Source: CAD feature listing. Evaluate the final solid. Frame: model axes, mm. A direction names the side the tool comes from. Round coordinates to 2 decimals unless told otherwise and drop trailing zeros. Loops run counter-clockwise (first coordinate to the right, second up) from the corner with the lowest first, then second, coordinate; pieces in that order, holes last. Notation, with made-up numbers: M 60.5,4.25 L 81.5,4.25 A14 cw 81.5,27.25 Z; hole C 2,33.5 d3. An arc over 180 degrees is marked long. Answer as a JSON object with one key per item and string values.
from build123d import *

# Parameters (mm, degrees)
F1_DEPTH = 6.35
F2_R     = 2.9845
F3_DEPTH = 6.35
F4_R     = 5.08
F5_R     = 3.81


with BuildPart() as f1:
    # F0 (on Top) → F1 (new body)
    with BuildSketch(Plane.XY):
        with BuildLine():
            Line((-10.9985226281, 6.35), (10.9985226281, 6.35))
            ThreePointArc((10.9985226281, 6.35), (0, 12.7), (-10.9985226281, 6.35))
        make_face()
        with BuildLine():
            ThreePointArc((-10.9985226281, -6.35), (-12.7, 0), (-10.9985226281, 6.35))
            Line((-10.9985226281, 6.35), (-31.75, 6.35))
            Line((-31.75, 6.35), (-31.75, -6.35))
            Line((-31.75, -6.35), (-10.9985226281, -6.35))
        make_face()
        with BuildLine():
            ThreePointArc((10.9985226281, -6.35), (12.2672579939, -3.2870018728), (12.7, 0))
            ThreePointArc((12.7, 0), (12.2672579939, 3.2870018728), (10.9985226281, 6.35))
            Line((10.9985226281, 6.35), (-10.9985226281, 6.35))
            ThreePointArc((-10.9985226281, 6.35), (-12.7, 0), (-10.9985226281, -6.35))
            Line((-10.9985226281, -6.35), (10.9985226281, -6.35))
        make_face()
        with BuildLine():
            ThreePointArc((10.9985226281, 6.35), (12.2672579939, 3.2870018728), (12.7, 0))
            ThreePointArc((12.7, 0), (12.2672579939, -3.2870018728), (10.9985226281, -6.35))
            Line((10.9985226281, -6.35), (31.75, -6.35))
            Line((31.75, -6.35), (31.75, 6.35))
            Line((31.75, 6.35), (10.9985226281, 6.35))
        make_face()
        with BuildLine():
            ThreePointArc((-10.9985226281, -6.35), (0, -12.7), (10.9985226281, -6.35))
            Line((10.9985226281, -6.35), (-10.9985226281, -6.35))
        make_face()
    extrude(amount=F1_DEPTH)

    # F2 (on face) → F3 (cut)
    with BuildSketch(Plane.XY.offset(6.35)):
        Circle(F2_R)
    extrude(amount=-F3_DEPTH, mode=Mode.SUBTRACT)

    # F4
    f4_edges = [f1.edges().sort_by_distance(p)[0] for p in [
        (-10.998523, 6.35, 3.175),
        (10.998523, -6.35, 3.175),
        (-10.998523, -6.35, 3.175),
        (10.998523, 6.35, 3.175),
    ]]
    fillet(f4_edges, radius=F4_R)

    # F5
    f5_edges = [f1.edges().sort_by_distance(p)[0] for p in [
        (-31.75, 6.35, 3.175),
        (-31.75, -6.35, 3.175),
        (31.75, -6.35, 3.175),
        (31.75, 6.35, 3.175),
    ]]
    fillet(f5_edges, radius=F5_R)


solid = f1.part
Item 1: Contact query for flat-ended pins moving along their axis: pin 1 Ø1.5 at (y, z) = (5.5, 4.5) entering from -X; pin 2 Ø1 at (x, y) = (-8, -9.5) entering from -Z; pin 3 Ø1 at (y, z) = (6, 4.5) entering from -X; pin 4 Ø3 at (x, z) = (15, 4.5) entering from +Y. Output: stop coordinate, or through.
Answer sheet:
{"pin 1": "stops at x = -31.04", "pin 2": "stops at z = 0", "pin 3": "stops at x = -30.34", "pin 4": "stops at y = 6.35"}
Item 2: Section A-A on z = 4.5. Return the cut outline in (x, y).
Answer sheet:
{"outline": "M -31.75,-2.54 A3.81 ccw -27.94,-6.35 L -13.62,-6.35 A5.08 cw -9.73,-8.16 A12.7 ccw 9.73,-8.16 A5.08 cw 13.62,-6.35 L 27.94,-6.35 A3.81 ccw 31.75,-2.54 L 31.75,2.54 A3.81 ccw 27.94,6.35 L 13.62,6.35 A5.08 cw 9.73,8.16 A12.7 ccw -9.73,8.16 A5.08 cw -13.62,6.35 L -27.94,6.35 A3.81 ccw -31.75,2.54 Z; hole C 0,0 d5.97"}
Item 3: Section C-C on y = 1.75. Return the cut outline in (x, z).
Answer sheet:
{"outline": "M -31.75,0 L -2.42,0 L -2.42,6.35 L -31.75,6.35 Z; M 2.42,0 L 31.75,0 L 31.75,6.35 L 2.42,6.35 Z"}
Item 4: Section B-B on x = 0. Return the cut outline in (y, z), then the cut area to 3 significant figures.
Answer sheet:
{"outline": "M -12.7,0 L -2.98,0 L -2.98,6.35 L -12.7,6.35 Z; M 2.98,0 L 12.7,0 L 12.7,6.35 L 2.98,6.35 Z", "area": "123 mm²"}
Item 5: Section D-D on x = -22. Return the cut outline in (y, z).
Answer sheet:
{"outline": "M -6.35,0 L 6.35,0 L 6.35,6.35 L -6.35,6.35 Z"}
Item 6: Line query: probe 1 along Y at (x, z) = (0, 2); probe 2 along Y at (x, z) = (-18, 3.5); probe 3 along Y at (x, z) = (1, 1.5). Output: solid intervals per line, ascending. Write a range as from..to.
Answer sheet:
{"probe 1": "y = -12.7..-2.98, 2.98..12.7", "probe 2": "y = -6.35..6.35", "probe 3": "y = -12.66..-2.81, 2.81..12.66"}
Item 7: Access query for faces 1 (the flat face through (-21, -6.35, 3)), 2 (the flat face through (21, -6.35, 3)), 3 (the flat face through (-21, 6.35, 3)), 4 (the flat face through (21, 6.35, 3)). Directions: +Z, -Z, +X, -X, +Y, -Y. A direction counts if a zero-diameter tool reaches every point of the face in a straight line with its end or side. Return the directions, or none.
Answer sheet:
{"face 1": "+Z, -Z, -X, -Y", "face 2": "+Z, -Z, +X, -Y", "face 3": "+Z, -Z, -X, +Y", "face 4": "+Z, -Z, +X, +Y"}
